Source: three-view drawing plus pictorial views. Frame: mm from the lowest corner of the part. A direction names the side the tool comes from. Coordinates: 2 decimals unless noted, no trailing zeros. Write each loop counter-clockwise with the first axis right and the second up, starting at its lowest first coordinate (ties: lowest second). Pieces come first, ordered by that corner, then holes. Notation, with made-up numbers: (51, -11.5) -> (88, -11.5) arc R21 ccw to (88, 8.5) -> close; hole circle Ø1 at (-36, 47). An arc over 180 degrees is marked (long way). One line per item, written item: value.
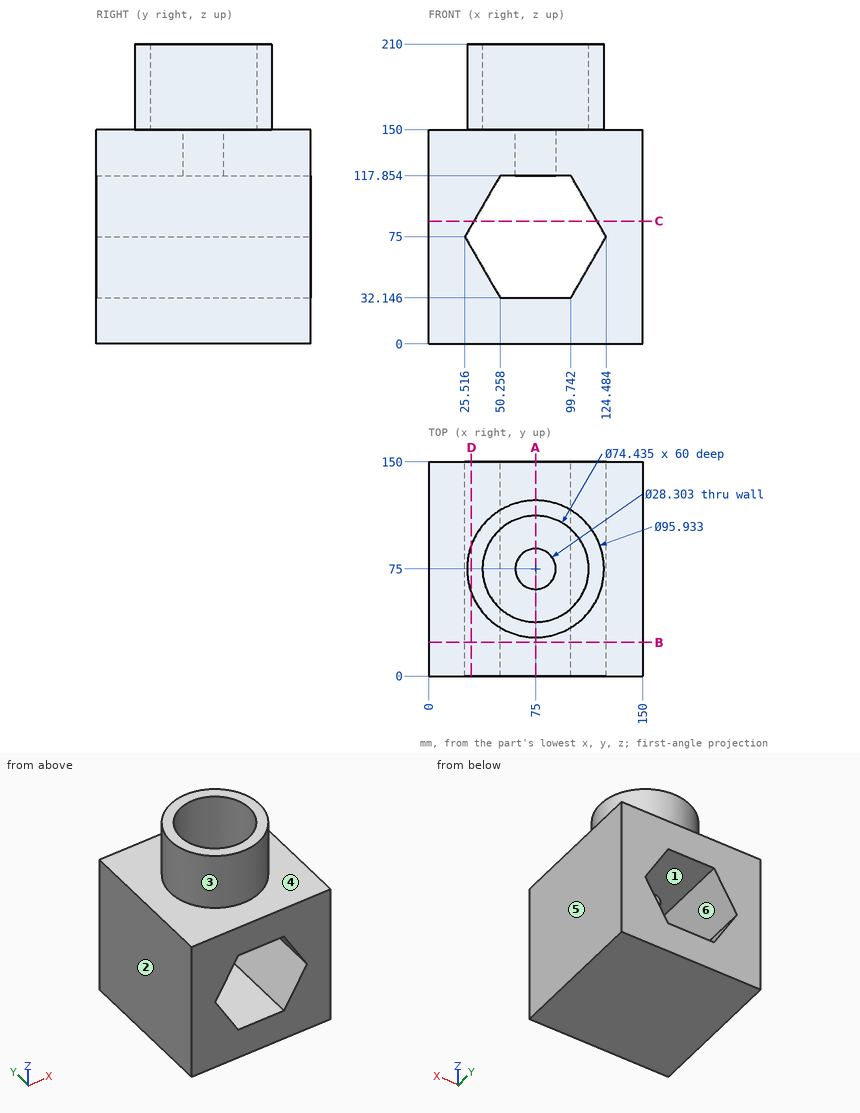
(1) Section D-D (x = 30). Return the cut outline in (y, z), then the cut area to 3 significant figures.
Responses:
outline: (0, 0) -> (150, 0) -> (150, 67.23) -> (0, 67.23) -> close; (0, 82.77) -> (150, 82.77) -> (150, 150) -> (91.61, 150) -> (91.61, 210) -> (58.39, 210) -> (58.39, 150) -> (0, 150) -> close
area: 22,200 mm2
(2) Section A-A (x = 75). Return the cut outline in (y, z) (1 decimal), then the cut area to 3 significant figures.
Responses:
outline: (0, 0) -> (150, 0) -> (150, 32.1) -> (0, 32.1) -> close; (0, 117.9) -> (60.8, 117.9) -> (60.8, 150) -> (37.8, 150) -> (37.8, 210) -> (27, 210) -> (27, 150) -> (0, 150) -> close; (89.2, 117.9) -> (150, 117.9) -> (150, 150) -> (123, 150) -> (123, 210) -> (112.2, 210) -> (112.2, 150) -> (89.2, 150) -> close
area: 10,000 mm2
(3) Section B-B (y = 23.5). Return the cut outline in (x, z) (1 decimal).
Responses:
outline: (0, 0) -> (150, 0) -> (150, 150) -> (0, 150) -> close; hole (25.5, 75) -> (50.3, 32.1) -> (99.7, 32.1) -> (124.5, 75) -> (99.7, 117.9) -> (50.3, 117.9) -> close
(4) Reachability of the marked faces 1, 2 and 3 from +Z, -Z, +X, -X, +Y, -Y: full face, straight path, thin tool, end or side. Return the list, or none.
Responses:
face 1: +Y, -Y
face 2: +Z, -Z, -X, +Y, -Y
face 3: +Z
(5) Section C-C (z = 86). Return the cut outline in (x, y), then the cut area to 3 significant figures.
Responses:
outline: (0, 0) -> (31.87, 0) -> (31.87, 150) -> (0, 150) -> close; (118.13, 0) -> (150, 0) -> (150, 150) -> (118.13, 150) -> close
area: 9,560 mm2
(6) First-contact query: pin 1 (6 mm diameter, centred on y = 108, z = 96, fed in from -X); pin 2 (24.5 mm diameter, centred on x = 86.5, y = 77.5, fed in from +Z); pin 3 (22.5 mm diameter, centred on x = 75, y = 75, fed in from +Z). Flat tips, straight axial feed; report the tip coordinate or a pass-through.
Responses:
pin 1: stops at x = 0
pin 2: stops at z = 150
pin 3: stops at z = 32.15
(7) Line query: line 1 (Y direction, x = 75, z = 186); line 2 (Z direction, x = 71, y = 97) (1 decimal); line 3 (Z direction, x = 64, y = 118.5) (1 decimal). Output: solid intervals per line, ascending. Write a range as [from, to].
Responses:
line 1: y = [27.03, 37.78], [112.22, 122.97]
line 2: z = [0, 32.1], [117.9, 150]
line 3: z = [0, 32.1], [117.9, 210]
(8) Pull-direction query (X, two-part tool) for the marked faces 4, 5 and 6; classes: released by +X, released by -X, zero draft, split by the parting line, or undercut.
Responses:
face 4: zero draft
face 5: released by +X
face 6: undercut
